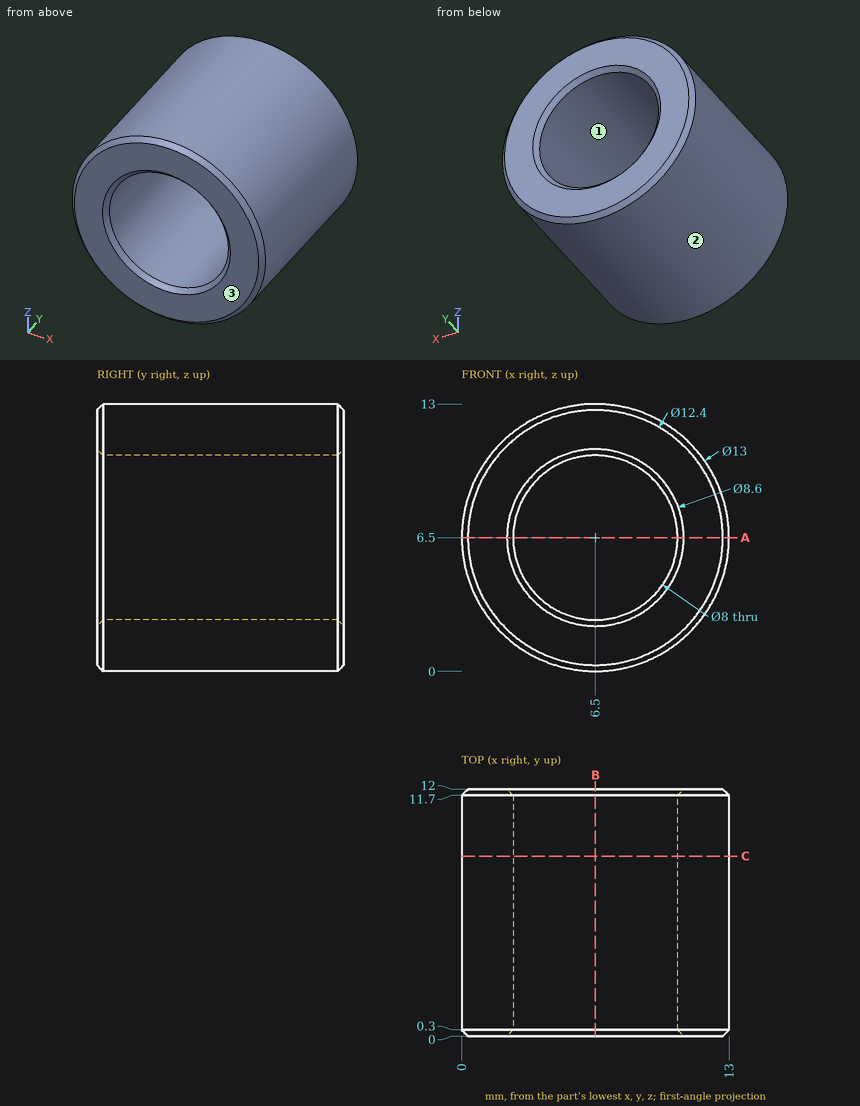
Study the drawing (mm; zero at the part's minimum x, y, z) and answer. Give positions to 0.01 mm unless a question says otherwise; leave off trailing zeros. Write each loop counter-clockwise with the first axis right and the second up, starting at its lowest first coordinate (ties: lowest second). Pieces come first, ordered by that corner, then holes.
Item 1: Section A-A, the plane z = 6.5 is taken. Write down the section's boundary in (x, y).
Item 2: Find the intervals of material crossed by line 1 along Z through (x, y) = (6.5, 3.5); line 2 along X through (y, z) = (4.25, 8); line 3 along X through (y, z) = (5.25, 9.25), in increasing order.
Item 3: Section B-B, the plane x = 6.5 is taken. Write down the section's boundary in (y, z).
Item 4: Section C-C, the plane y = 8.75 is taken. Write down the section's boundary in (x, z).
Item 5: Flat-ended cylindrical pins translate along their axes: P1, Ø2, axis at y = 4, z = 10.5, coming from the -X side; P2, Ø3, axis at x = 1.5, z = 5, coming from the -Y side; P3, Ø1.5, axis at x = 9.5, y = 2.5, coming from the -Z side; P4, Ø1.5, axis at y = 1.5, z = 11, coming from the +X side. Find the tip coordinate at first contact, or state that the pin passes through.
Item 6: Determine the mould class of the marked faces 1, 2 and 3 for opening direction X: released by +X, released by -X, zero draft, split by the parting line, or undercut.
Completed:
1. outline: (0, 0.3) - (0.3, 0) - (2.2, 0) - (2.5, 0.3) - (2.5, 11.7) - (2.2, 12) - (0.3, 12) - (0, 11.7) - close; (10.5, 0.3) - (10.8, 0) - (12.7, 0) - (13, 0.3) - (13, 11.7) - (12.7, 12) - (10.8, 12) - (10.5, 11.7) - close
2. line 1: z = 0 to 2.5, 10.5 to 13
2. line 2: x = 0.18 to 2.79, 10.21 to 12.82
2. line 3: x = 0.61 to 3.6, 9.4 to 12.39
3. outline: (0, 0.3) - (0.3, 0) - (11.7, 0) - (12, 0.3) - (12, 2.2) - (11.7, 2.5) - (0.3, 2.5) - (0, 2.2) - close; (0, 10.8) - (0.3, 10.5) - (11.7, 10.5) - (12, 10.8) - (12, 12.7) - (11.7, 13) - (0.3, 13) - (0, 12.7) - close
4. outline: circle Ø13 at (6.5, 6.5); hole circle Ø8 at (6.5, 6.5)
5. P1: stops at x = 0.73
5. P2: stops at y = 0
5. P3: stops at z = 0.4
5. P4: stops at x = 11.81
6. face 1: undercut
6. face 2: split by the parting line
6. face 3: zero draft
